Could you check a few things on this model? Use its own coordinates, in mm. Face numbers are marked on the shaded views. Give positions to 0.01 mm unless a question says otherwise; leave off trailing zeros. Order: outer loops, then holes, each group sorted by start corner. A loop starts at its lowest first (then second) coordinate and runs counter-clockwise, first axis right, second up. Notation, with made-up numbers: (-5.75, -8) - (12.25, -8) arc R15 ccw to (12.25, 16) - close; hole circle Ø8 at (-31.75, 48.25). An arc over 180 degrees is marked (long way). Put each result on its own line as item: value.
from build123d import *

# Parameters (mm, degrees)
F0_R     = 3.2385
F1_DEPTH = 2.1082
F1_TAPER = 41
F3_DEPTH = 5.8293
F5_DEPTH = 1.27


with BuildPart() as f1:
    # F0 (on Top) → F1 (new body)
    with BuildSketch(Plane.XY):
        Circle(F0_R)
    extrude(amount=-F1_DEPTH, taper=F1_TAPER)

    # F3 (add, through all): a face of the model
    f3_faces = [f1.faces().sort_by_distance(p)[0] for p in [
        (0, 0, -2.1082),
    ]]
    extrude(f3_faces, amount=F3_DEPTH)

    # F4 (on face) → F5 (cut)
    with BuildSketch(Plane.XY):
        Polygon((0.79375, -0.4582717762), (0.79375, 0.4582717762), (0, 0.9165435523), (-0.79375, 0.4582717762), (-0.79375, -0.4582717762), (0, -0.9165435523), align=None)
    extrude(amount=-F5_DEPTH, mode=Mode.SUBTRACT)


solid = f1.part
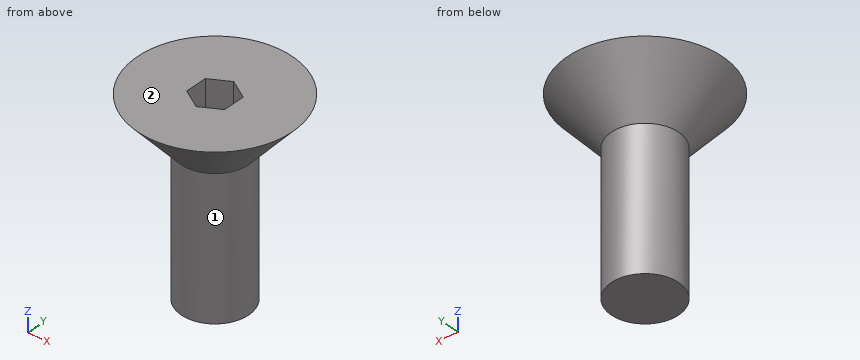
1) We'd pull the mould along Y, two halves only. Please class the marked faces 1 and 2: pulls with the +Y half, pulls with the -Y half, needs draft (parallel to the pull), parting line crosses it, or undercut.
Filled in:
face 1: parting line crosses it
face 2: needs draft
2) Suppose I cut it at A-A, the plane z = -5.5. List the corners of the cut face in (x, y) for me.
Filled in:
outline: circle Ø2.81 at (0, 0)
3) Suppose I cut it at B-B, the plane z = -1.5. List the corners of the cut face in (x, y) for me, and give its area (3 significant figures).
Filled in:
outline: circle Ø3.87 at (0, 0)
area: 11.8 mm^2
4) If I drill on line 1 (Z direction, x = 3, y = -0.5); line 2 (Y direction, x = -0.25, z = -4); line 3 (X direction, y = -1, z = -3.5), over which ranges is the centre line in solid material (lowest first)? Write a range as [from, to].
Filled in:
line 1: z = [-0.23, 0]
line 2: y = [-1.38, 1.38]
line 3: x = [-0.99, 0.99]
5) I'm going to push flat-ended pins straight in: pin 1 (1 mm diameter, centred on y = 0, z = -1, fed in from +X); pin 2 (2 mm diameter, centred on y = 2, z = -2, fed in from -X); pin 3 (1 mm diameter, centred on x = 2.5, y = 0.5, fed in from -Z). Where does each tip first touch, or does it pass through?
Filled in:
pin 1: stops at x = 2.8
pin 2: stops at x = -1.69
pin 3: stops at z = -1.37
